Source: CAD feature listing. Evaluate the final solid. Frame: model axes, mm. A direction names the side the tool comes from. Give positions to 0.01 mm unless a question says otherwise; leave off trailing zeros. Order: outer loops, then holes, each group sorted by start corner. A loop starts at its lowest first (then second) coordinate and runs counter-clockwise, first axis right, second up. Notation, with made-up numbers: M -3,36.5 L 40,36.5 A21 ccw 40,58.5 Z; hole C 29.25,61 d9. An arc over 180 degrees is marked long. Return JSON: item names as keys, results as strings.
from build123d import *

# Parameters (mm, degrees)
PLASTIC_DEPTH   = 2.54
CONTACT_DEPTH   = 0.3
CHAMFER1_SIZE   = 0.1
LPATTERN1_COUNT = 7
LPATTERN1_PITCH = 2.54


with BuildPart() as part:
    # Sketch1 → Plastic (new body)
    with BuildSketch(Plane(origin=(0, 0, 0), x_dir=(0, 0, -1), z_dir=(1, 0, 0))):
        Polygon((-2.04, 1.27), (-0.5, 1.27), (0, 0.77), (0, -0.77), (-0.5, -1.27), (-2.04, -1.27), (-2.54, -0.77), (-2.54, 0.77), align=None)
    extrude(amount=PLASTIC_DEPTH)

    # Sketch2 → Contact (add, symmetric)
    with BuildSketch(Plane(origin=(0, 0, 0), x_dir=(1, 0, 0), z_dir=(0, 1, 0))):
        with BuildLine():
            Line((-1.86, 3.36), (-1.86, -0.67))
            ThreePointArc((-1.86, -0.67), (-1.596396103, -1.306396103), (-0.96, -1.57))
            Line((-0.96, -1.57), (8.9, -1.57))
            Line((8.9, -1.57), (8.9, -0.97))
            Line((8.9, -0.97), (-0.96, -0.97))
            ThreePointArc((-0.96, -0.97), (-1.172132034, -0.882132034), (-1.26, -0.67))
            Line((-1.26, -0.67), (-1.26, 3.36))
            Line((-1.26, 3.36), (-1.86, 3.36))
        make_face()
    extrude(amount=CONTACT_DEPTH, both=True)

    # Chamfer1
    chamfer1_edges = [part.edges().sort_by_distance(p)[0] for p in [
        (8.9, 0, 0.97),
        (8.9, 0.3, 1.27),
        (-1.56, -0.3, -3.36),
        (-1.26, 0, -3.36),
        (-1.86, 0, -3.36),
        (8.9, -0.3, 1.27),
        (8.9, 0, 1.57),
        (-1.56, 0.3, -3.36),
    ]]
    chamfer(chamfer1_edges, length=CHAMFER1_SIZE)

    # LPattern1: part ×7


with BuildPart() as part_1:
    add(part.part)
    with Locations(*[(0, i * LPATTERN1_PITCH, 0) for i in range(1, LPATTERN1_COUNT)]):
        add(part.part)


solid = part_1.part
1. Section query B-B (x = 5.5). Return loops of the section in (y, z), then the cut area to 3 significant figures.
Evaluation:
{"outline": "M -0.3,0.97 L 0.3,0.97 L 0.3,1.57 L -0.3,1.57 Z; M 2.24,0.97 L 2.84,0.97 L 2.84,1.57 L 2.24,1.57 Z; M 4.78,0.97 L 5.38,0.97 L 5.38,1.57 L 4.78,1.57 Z; M 7.32,0.97 L 7.92,0.97 L 7.92,1.57 L 7.32,1.57 Z; M 9.86,0.97 L 10.46,0.97 L 10.46,1.57 L 9.86,1.57 Z; M 12.4,0.97 L 13,0.97 L 13,1.57 L 12.4,1.57 Z; M 14.94,0.97 L 15.54,0.97 L 15.54,1.57 L 14.94,1.57 Z", "area": "2.52 mm^2"}
2. Section query D-D (z = 1.85). Return loops of the section in (x, y), then the cut area to 3 significant figures.
Evaluation:
{"outline": "M 0,-1.27 L 2.54,-1.27 L 2.54,16.51 L 0,16.51 Z", "area": "45.2 mm^2"}
3. Ray query, probe 1 along Z at (x, y) = (1.25, 5.5); probe 2 along X at (y, z) = (10.25, -0.05); probe 3 along Z at (x, y) = (5.5, -0.25). Return the intervals inside material, ascending.
Evaluation:
{"probe 1": "z = 0 to 2.54", "probe 2": "x = -1.86 to -1.26", "probe 3": "z = 0.97 to 1.57"}
4. Set-up query: faces 5 (the face through (1, 10, 0)), 6 (the face through (-1.6, 0.3, -0.3)), 7 (the face through (1, 15, 2.54)). Return all of +Z, -Z, +X, -X, +Y, -Y with unobstructed straight access to the full face (end or side cutting, diameter ignored); none if empty.
Evaluation:
{"face 5": "-Z, +X, +Y, -Y", "face 6": "+Z, -Z, -X", "face 7": "+Z, +X, -X, +Y, -Y"}
5. Section query C-C (y = 4.5). Return loops of the section in (x, z), then the cut area to 3 significant figures.
Evaluation:
{"outline": "M 0,0 L 2.54,0 L 2.54,2.54 L 0,2.54 Z", "area": "6.45 mm^2"}
6. Draft query along Y for faces 1 (the face through (-1.6, -0.3, -0.3)), 2 (the face through (-1.6, 12.4, -0.3)), 3 (the face through (-1.6, 2.5, 1.3)), 4 (the face through (2.54, 7.7, 0.7)). Return one class per face: pulls with the +Y half, pulls with the -Y half, needs draft (parallel to the pull), parting line crosses it, or undercut.
Evaluation:
{"face 1": "pulls with the -Y half", "face 2": "undercut", "face 3": "needs draft", "face 4": "undercut"}
7. Section query A-A (z = -1.15). Return loops of the section in (x, y), then the cut area to 3 significant figures.
Evaluation:
{"outline": "M -1.86,-0.3 L -1.26,-0.3 L -1.26,0.3 L -1.86,0.3 Z; M -1.86,2.24 L -1.26,2.24 L -1.26,2.84 L -1.86,2.84 Z; M -1.86,4.78 L -1.26,4.78 L -1.26,5.38 L -1.86,5.38 Z; M -1.86,7.32 L -1.26,7.32 L -1.26,7.92 L -1.86,7.92 Z; M -1.86,9.86 L -1.26,9.86 L -1.26,10.46 L -1.86,10.46 Z; M -1.86,12.4 L -1.26,12.4 L -1.26,13 L -1.86,13 Z; M -1.86,14.94 L -1.26,14.94 L -1.26,15.54 L -1.86,15.54 Z", "area": "2.52 mm^2"}
8. First-contact query: pin 1 (0.7 mm diameter, centred on x = 7, z = 1.5, fed in from -Y); pin 2 (1.7 mm diameter, centred on x = 1, y = 13, fed in from -Z); pin 3 (0.5 mm diameter, centred on x = 6, z = 1, fed in from +Y); pin 4 (2 mm diameter, centred on x = 0, z = -2, fed in from +Y). Flat tips, straight axial feed; report the tip coordinate or a pass-through.
Evaluation:
{"pin 1": "stops at y = -0.3", "pin 2": "stops at z = 0", "pin 3": "stops at y = 15.54", "pin 4": "passes through"}
